The model under review builds one solid part; all positions refer to its coordinate system, in mm. A direction names the side the tool comes from. Coordinates: 2 decimals unless noted, no trailing zeros. Order: outer loops, then holes, each group sorted by start corner. A loop starts at its lowest first (then second) coordinate and runs counter-clockwise, first axis right, second up.
```python
from build123d import *

# Parameters (mm, degrees)
F2_DEPTH = 482.6
F5_DEPTH = 95.25
F6_DEPTH = 457.2
F7_W     = 391.6691155402
F7_H     = 457.2
F8_DEPTH = 38.1


with BuildPart() as f2:
    # F1 (on face) → F2 (new body)
    with BuildSketch(Plane.XY):
        Polygon((848.8691155402, -187.3188240631), (677.4191155402, 263.7994060052), (105.9191155402, 263.7994060052), (-65.5308844598, -187.3188240631), align=None)
    extrude(amount=F2_DEPTH)

    # F3 (on face) → F5 (join)
    with BuildSketch(Plane.XY.offset(482.6)):
        Polygon((677.4191155402, 263.7994060052), (105.9191155402, 263.7994060052), (-65.5308844598, -187.3188240631), (848.8691155402, -187.3188240631), align=None)
        Polygon((1.5293506387, -149.2188240631), (144.0191155402, 225.6994060052), (639.3191155402, 225.6994060052), (781.8088804417, -149.2188240631), align=None, mode=Mode.SUBTRACT)
        Polygon((639.3191155402, 225.6994060052), (144.0191155402, 225.6994060052), (1.5293506387, -149.2188240631), (781.8088804417, -149.2188240631), align=None)
    extrude(amount=F5_DEPTH)

    # F4 (on face) → F6 (cut)
    with BuildSketch(Plane.XY.offset(482.6)):
        Polygon((781.8088804417, -149.2188240631), (639.3191155402, 225.6994060052), (144.0191155402, 225.6994060052), (1.5293506387, -149.2188240631), align=None)
    extrude(amount=-F6_DEPTH, mode=Mode.SUBTRACT)

    # F7 (on face) → F8 (cut)
    with BuildSketch(Plane.XZ.offset(187.3188240631)):
        with Locations((587.5036733103, 254)):
            Rectangle(F7_W, F7_H)
        with Locations((195.8345577701, 254)):
            Rectangle(F7_W, F7_H)
    extrude(amount=-F8_DEPTH, mode=Mode.SUBTRACT)


solid = f2.part
```
(1) Draft analysis for pull direction Z (two halves, no side actions). For faces 3 (the face through (386, 16, 25.4)), 4 (the face through (385, 41, 577.85)), 5 (the face through (397, 16, 482.6)), 6 (the face through (21.394, 41.398, 284.88)), state which applies: released by +Z, released by -Z, zero draft, split by the parting line, or undercut.
A:
face 3: undercut
face 4: released by +Z
face 5: undercut
face 6: zero draft
(2) We need section B-B, the plane x = 195.5. Write out the cut boundary in (y, z).
A:
outline: (-187.32, 0) - (263.8, 0) - (263.8, 577.85) - (-187.32, 577.85) - (-187.32, 482.6) - (225.7, 482.6) - (225.7, 25.4) - (-187.32, 25.4) - close
(3) We need section C-C, the plane y = 100. Write out the cut boundary in (x, z).
A:
outline: (43.67, 0) - (739.67, 0) - (739.67, 577.85) - (43.67, 577.85) - close; hole (96.25, 25.4) - (687.09, 25.4) - (687.09, 482.6) - (96.25, 482.6) - close
(4) For pin 1 Ø1.7 at (x, z) = (1, 363) entering from -Y; pin 2 Ø3 at (y, z) = (213.5, 417) entering from +X; pin 3 Ø10 at (y, z) = (-25.5, 430) entering from +X, all flat-tipped, find the tip position at first contact; note any pin that passes through.
A:
pin 1: stops at y = -149.22
pin 2: stops at x = 697.11
pin 3: stops at x = 789.27
(5) We need section A-A, the plane z = 334. Write out the cut boundary in (x, y), and give its area (3 significant figures).
A:
outline: (-65.53, -187.32) - (0, -187.32) - (0, -149.22) - (1.53, -149.22) - (144.02, 225.7) - (639.32, 225.7) - (781.81, -149.22) - (783.34, -149.22) - (783.34, -187.32) - (848.87, -187.32) - (677.42, 263.8) - (105.92, 263.8) - close
area: 66,200 mm2
(6) Machinability: for faces 1 (the face through (395, 225.699, 257)), 2 (the face through (396, 263.799, 285)), which of the approach directions +Z, -Z, +X, -X, +Y, -Y give a long, thin tool a straight path to every point of the face, cutting with its end or side? Answer none if there is none.
A:
face 1: -Y
face 2: +Z, -Z, +X, -X, +Y
(7) We need section D-D, the plane y = -15. Write out the cut boundary in (x, z).
A:
outline: (-0.04, 0) - (783.38, 0) - (783.38, 577.85) - (-0.04, 577.85) - close; hole (52.54, 25.4) - (730.8, 25.4) - (730.8, 482.6) - (52.54, 482.6) - close
(8) Wall thickness on probe 1 along Z at (x, y) = (625.5, -92); probe 2 along Y at (x, z) = (262, 113.5); probe 3 along X at (y, z) = (-168, 255): over which ranges is each line inside the solid? List them lowest first.
A:
probe 1: z = 0 to 25.4, 482.6 to 577.85
probe 2: y = 225.7 to 263.8
probe 3: x = -58.19 to 0, 783.34 to 841.53
